```python
from build123d import *

# Parameters (mm, degrees)
BOSS_EXTRUDE1_DEPTH = 6.35
SKETCH2_R           = 1.4224
BOSS_EXTRUDE2_DEPTH = 4.7625
SKETCH7_R           = 1.4224
CUT_EXTRUDE4_DEPTH  = 4.7625


with BuildPart() as part:
    # Sketch1 → Boss-Extrude1 (new body)
    with BuildSketch(Plane(origin=(0, 0, 0), x_dir=(1, 0, 0), z_dir=(0, 1, 0))):
        Polygon((-2.38125, 1.374815329), (-2.38125, -1.374815329), (0, -2.749630657), (2.38125, -1.374815329), (2.38125, 1.374815329), (0, 2.749630657), align=None)
    extrude(amount=BOSS_EXTRUDE1_DEPTH)

    # Sketch2 → Boss-Extrude2 (add)
    with BuildSketch(Plane(origin=(0, 6.35, 0), x_dir=(1, 0, 0), z_dir=(0, 1, 0))):
        Circle(SKETCH2_R)
    extrude(amount=BOSS_EXTRUDE2_DEPTH)

    # Sketch7 → Cut-Extrude4 (cut)
    with BuildSketch(Plane.XZ):
        Circle(SKETCH7_R)
    extrude(amount=-CUT_EXTRUDE4_DEPTH, mode=Mode.SUBTRACT)


solid = part.part
```
Can you work these out from the model? Positions are in its coordinate system, mm. A direction names the side the tool comes from. Round coordinates to 2 decimals unless told otherwise and drop trailing zeros. Order: outer loops, then holes, each group sorted by start corner. A loop starts at its lowest first (then second) coordinate and runs counter-clockwise, first axis right, second up. Notation, with made-up numbers: (20.5, 4.25) -> (38.5, 4.25) arc R26 cw to (38.5, 32.25) -> close; hole circle Ø9 at (77.5, 73.5). An arc over 180 degrees is marked (long way). Return JSON: item names as keys, results as strings. Group by question number.
1. If we section it at D-D, the plane x = 1.05: Write out the boundary of the cut face in (y, z).
2. Will these pins go through, and if not, where does the flat tip stop? pin 1 (1 mm diameter, centred on x = -1.5, z = 1, fed in from -Y); pin 2 (2 mm diameter, centred on x = -2, z = -2, fed in from +Y); pin 3 (2 mm diameter, centred on x = -0.5, y = 9.5, fed in from +Z).
3. If we section it at B-B, the plane z = 0: Write out the boundary of the cut face in (x, y).
4. We'd pull the mould along X, two halves only. Please class faces 1 (the face through (1.21, 3.13, -2.05)), 2 (the face through (-0.31, 2.35, -1.39)), 3 (the face through (-2.381, 3, 0)), 4 (the face through (-1.1, 0, 1.2)): released by +X, released by -X, zero draft, split by the parting line, or undercut.
5. If we section it at A-A, the plane y = 2.75: Write out the boundary of the cut face in (x, z).
6. If we section it at C-C, the plane y = 8: Write out the boundary of the cut face in (x, z), then the cut area to 3 significant figures.
7. I need wall thicknesses on line 1 (Y direction, x = 0.4, z = -1.8); line 2 (Y direction, x = 0.5, z = -0.15); line 3 (Z direction, x = -0.2, y = 2). Which ranges of each line are inside material? Lowest first, please. Write a range as [from, to].
8. Which directions (+Z, -Z, +X, -X, +Y, -Y) give clear straight access to the entire face, cutting with the end or side of a thin tool? Please do faces 5 (the face through (-0.31, 8.7, 1.39)), 6 (the face through (-1.21, 3.13, 2.05)), 7 (the face through (0, 4.762, 0)).
Output values:
{
 "1": {"outline": "(0, -2.14) -> (6.35, -2.14) -> (6.35, -0.96) -> (11.11, -0.96) -> (11.11, 0.96) -> (6.35, 0.96) -> (6.35, 2.14) -> (0, 2.14) -> (0, 0.96) -> (4.76, 0.96) -> (4.76, -0.96) -> (0, -0.96) -> close"},
 "2": {"pin 1": "y = 0", "pin 2": "y = 6.35", "pin 3": "z = 1.42"},
 "3": {"outline": "(-2.38, 0) -> (-1.42, 0) -> (-1.42, 4.76) -> (1.42, 4.76) -> (1.42, 0) -> (2.38, 0) -> (2.38, 6.35) -> (1.42, 6.35) -> (1.42, 11.11) -> (-1.42, 11.11) -> (-1.42, 6.35) -> (-2.38, 6.35) -> close"},
 "4": {"face 1": "released by +X", "face 2": "undercut", "face 3": "released by -X", "face 4": "zero draft"},
 "5": {"outline": "(-2.38, -1.37) -> (0, -2.75) -> (2.38, -1.37) -> (2.38, 1.37) -> (0, 2.75) -> (-2.38, 1.37) -> close; hole circle Ø2.84 at (0, 0)"},
 "6": {"outline": "circle Ø2.84 at (0, 0)", "area": "6.36 mm²"},
 "7": {"line 1": "[0, 6.35]", "line 2": "[4.76, 11.11]", "line 3": "[-2.63, -1.41], [1.41, 2.63]"},
 "8": {"face 5": "+Y", "face 6": "+Z, -X, +Y, -Y", "face 7": "-Y"}
}
